Verification items for the finished model (mm, model axes). A direction names the side the tool comes from. Coordinates: 2 decimals unless noted, no trailing zeros. Order: outer loops, then holes, each group sorted by start corner. A loop starts at its lowest first (then second) coordinate and runs counter-clockwise, first axis right, second up. Notation, with made-up numbers: (17, -38) -> (64, -38) arc R16 cw to (64, -32) -> close; hole circle Ø7 at (-7.75, 74.25). An arc over 180 degrees is marked (long way). Write item = value, one per line. Start each with the question number.
from build123d import *

# Parameters (mm, degrees)
SKETCH1_W           = 94
SKETCH1_H           = 32
BOSS_EXTRUDE1_DEPTH = 4
CAVITY1_START       = 5
CAVITY1_OUTLINE_W   = 2
CAVITY1_OUTLINE_H   = 5.8
CAVITY1_DEPTH       = 84.5
CAVITY1_START_2     = 73.85
CAVITY1_2_OUTLINE_W = 2
CAVITY1_2_OUTLINE_H = 10.4
CAVITY1_2_DEPTH     = 15.65
CAVITY1_START_3     = 59.35
CAVITY1_3_OUTLINE_W = 2
CAVITY1_3_OUTLINE_H = 2.3
CAVITY1_3_DEPTH     = 14.5
CAVITY1_4_OUTLINE_W = 2
CAVITY1_4_OUTLINE_H = 10.4
CAVITY1_4_DEPTH     = 5.35
CAVITY1_START_4     = 16.15
CAVITY1_5_OUTLINE_W = 2
CAVITY1_5_OUTLINE_H = 10.4
CAVITY1_5_DEPTH     = 5
CAVITY1_START_5     = 26.95
CAVITY1_6_OUTLINE_W = 2
CAVITY1_6_OUTLINE_H = 10.4
CAVITY1_6_DEPTH     = 5
CAVITY1_START_6     = 37.75
CAVITY1_7_OUTLINE_W = 2
CAVITY1_7_OUTLINE_H = 10.4
CAVITY1_7_DEPTH     = 5
CAVITY1_START_7     = 48.55
CAVITY1_8_OUTLINE_W = 2
CAVITY1_8_OUTLINE_H = 10.4
CAVITY1_8_DEPTH     = 5
CAVITY1_9_OUTLINE_W = 2
CAVITY1_9_OUTLINE_H = 5.8
CAVITY1_9_DEPTH     = 5


# Read off the part's stored shape, not the designer's step: Cavity1
with BuildPart() as part:
    # Sketch1 → Boss-Extrude1 (new body)
    with BuildSketch(Plane(origin=(0, 0, 0), x_dir=(1, 0, 0), z_dir=(0, 1, 0))):
        with Locations((47, 16)):
            Rectangle(SKETCH1_W, SKETCH1_H)
    extrude(amount=BOSS_EXTRUDE1_DEPTH)

    # Cavity1 outline → Cavity1 (cut)
    with BuildSketch(Plane.YZ.offset(CAVITY1_START)):
        with Locations((3, -7.9)):
            Rectangle(CAVITY1_OUTLINE_W, CAVITY1_OUTLINE_H)
        with Locations((3, -24.1)):
            Rectangle(CAVITY1_OUTLINE_W, CAVITY1_OUTLINE_H)
    extrude(amount=CAVITY1_DEPTH, mode=Mode.SUBTRACT)

    # Cavity1 2 outline → Cavity1 2 (cut)
    with BuildSketch(Plane.YZ.offset(CAVITY1_START_2)):
        with Locations((3, -16)):
            Rectangle(CAVITY1_2_OUTLINE_W, CAVITY1_2_OUTLINE_H)
    extrude(amount=CAVITY1_2_DEPTH, mode=Mode.SUBTRACT)

    # Cavity1 3 outline → Cavity1 3 (cut)
    with BuildSketch(Plane.YZ.offset(CAVITY1_START_3)):
        with Locations((3, -11.95)):
            Rectangle(CAVITY1_3_OUTLINE_W, CAVITY1_3_OUTLINE_H)
        with Locations((3, -20.05)):
            Rectangle(CAVITY1_3_OUTLINE_W, CAVITY1_3_OUTLINE_H)
    extrude(amount=CAVITY1_3_DEPTH, mode=Mode.SUBTRACT)

    # Cavity1 4 outline → Cavity1 4 (cut)
    with BuildSketch(Plane.YZ.offset(CAVITY1_START)):
        with Locations((3, -16)):
            Rectangle(CAVITY1_4_OUTLINE_W, CAVITY1_4_OUTLINE_H)
    extrude(amount=CAVITY1_4_DEPTH, mode=Mode.SUBTRACT)

    # Cavity1 5 outline → Cavity1 5 (cut)
    with BuildSketch(Plane.YZ.offset(CAVITY1_START_4)):
        with Locations((3, -16)):
            Rectangle(CAVITY1_5_OUTLINE_W, CAVITY1_5_OUTLINE_H)
    extrude(amount=CAVITY1_5_DEPTH, mode=Mode.SUBTRACT)

    # Cavity1 6 outline → Cavity1 6 (cut)
    with BuildSketch(Plane.YZ.offset(CAVITY1_START_5)):
        with Locations((3, -16)):
            Rectangle(CAVITY1_6_OUTLINE_W, CAVITY1_6_OUTLINE_H)
    extrude(amount=CAVITY1_6_DEPTH, mode=Mode.SUBTRACT)

    # Cavity1 7 outline → Cavity1 7 (cut)
    with BuildSketch(Plane.YZ.offset(CAVITY1_START_6)):
        with Locations((3, -16)):
            Rectangle(CAVITY1_7_OUTLINE_W, CAVITY1_7_OUTLINE_H)
    extrude(amount=CAVITY1_7_DEPTH, mode=Mode.SUBTRACT)

    # Cavity1 8 outline → Cavity1 8 (cut)
    with BuildSketch(Plane.YZ.offset(CAVITY1_START_7)):
        with Locations((3, -16)):
            Rectangle(CAVITY1_8_OUTLINE_W, CAVITY1_8_OUTLINE_H)
    extrude(amount=CAVITY1_8_DEPTH, mode=Mode.SUBTRACT)

    # Cavity1 9 outline → Cavity1 9 (cut)
    with BuildSketch(Plane.YZ.offset(CAVITY1_START_3)):
        with Locations((3, -16)):
            Rectangle(CAVITY1_9_OUTLINE_W, CAVITY1_9_OUTLINE_H)
    extrude(amount=CAVITY1_9_DEPTH, mode=Mode.SUBTRACT)


solid = part.part
Item 1: Section check A-A (y = 3.4). State how many separate pieces and enclosed holes the cut face has, then the cut area to 3 significant figures.
Item 2: Thickness scan on line 1 (Z direction, x = 48, y = 2.7); line 2 (Z direction, x = 76.5, y = 3.8); line 3 (Z direction, x = 72, y = 3.25). Record the ranges inside material, lowest first.
Item 3: Section check D-D (x = 83). Record the boundary of the cut face in (y, z), then the cut area to 3 significant figures.
Item 4: Section check C-C (z = -9.5). Record the boundary of the cut face in (x, y).
Item 5: Mould release check, pull along Z, two halves, no side actions. Record for faces 3 (the flat face through (13, 4, -16)), 4 (the flat face through (46, 2, 0)), 5 (the flat face through (53.55, 3, -16)): pulls with the +Z half, pulls with the -Z half, needs draft (parallel to the pull), parting line crosses it, or undercut.
Item 6: Gauge pin test, flat end, axial feed: P1, Ø2, axis at x = 63, z = -19.5, coming from the +Y side. Record the tip position at first contact, or that the pin passes through.
Item 7: Tool access check on faces 1 (the flat face through (47, 4, -28)), 2 (the flat face through (47, 3, -27)). Record the directions out of +Z, -Z, +X, -X, +Y, -Y that give a thin tool (end or side, any length) a straight path to the whole face; none if there is none.
Item 8: Section check B-B (x = 24.5). Record the boundary of the cut face in (y, z).
Filled sheet:
q1.separate_pieces = 7
q1.enclosed_holes = 1
q1.area = 1,510 mm^2
q2.line_1 = -32 to -27, -21.2 to -10.8, -5 to 0
q2.line_2 = -32 to -27, -5 to 0
q2.line_3 = -32 to -27, -18.9 to -13.1, -5 to 0
q3.outline = (0, -32) -> (4, -32) -> (4, -27) -> (2, -27) -> (2, -5) -> (4, -5) -> (4, 0) -> (0, 0) -> close
q3.area = 84.0 mm^2
q4.outline = (0, 0) -> (94, 0) -> (94, 4) -> (89.5, 4) -> (89.5, 2) -> (5, 2) -> (5, 4) -> (0, 4) -> close
q5.face_3 = needs draft
q5.face_4 = pulls with the +Z half
q5.face_5 = undercut
q6.P1 = 2
q7.face_1 = +Z, -Z, +X, -X, +Y
q7.face_2 = +Y
q8.outline = (0, -32) -> (4, -32) -> (4, -27) -> (2, -27) -> (2, -21.2) -> (4, -21.2) -> (4, -10.8) -> (2, -10.8) -> (2, -5) -> (4, -5) -> (4, 0) -> (0, 0) -> close
